Could you check a few things on this model? Use its own coordinates, in mm. Round coordinates to 2 decimals unless told otherwise and drop trailing zeros. Write each loop counter-clockwise with the first axis right and the second up, starting at its lowest first coordinate (ties: lowest second). Pieces come first, ordered by that corner, then holes. Notation, with made-up numbers: (11, 12.5) -> (36, 12.5) arc R20 cw to (36, 19.5) -> close; hole circle Ø11 at (14, -1.5). An arc over 180 degrees is marked (long way). Answer in a Markdown table with one row per item.
from build123d import *

# Parameters (mm, degrees)
END_STOP_SHEET_SKETCH_W                   = 2
END_STOP_SHEET_SKETCH_H                   = 54
END_STOP_SHEET_DEPTH                      = 11
SCREW_END_CLEARANCE_SKETCH_R              = 3.4
SCREW_END_CLEARANCE_DEPTH                 = 2.2
M3_COUNTERSUNK_CLEARANCE_1_BORE_PROFILE_R = 1.7
M3_COUNTERSUNK_CLEARANCE_1_BORE_DEPTH     = 2.2
M3_COUNTERSUNK_CLEARANCE_2_BORE_PROFILE_R = 1.7
M3_COUNTERSUNK_CLEARANCE_2_BORE_DEPTH     = 2.2


with BuildPart() as part:
    # End stop sheet sketch → End stop sheet (new body)
    with BuildSketch(Plane.XY.offset(-33.5)):
        with Locations((59.2, -27.5)):
            Rectangle(END_STOP_SHEET_SKETCH_W, END_STOP_SHEET_SKETCH_H)
    extrude(amount=END_STOP_SHEET_DEPTH)

    # Screw end clearance sketch → Screw end clearance (cut)
    with BuildSketch(Plane(origin=(58.1, 0, 0), x_dir=(0, 0, -1), z_dir=(1, 0, 0))):
        with Locations((19.5, -29)):
            Circle(SCREW_END_CLEARANCE_SKETCH_R)
    extrude(amount=SCREW_END_CLEARANCE_DEPTH, mode=Mode.SUBTRACT)

    # M3 countersunk clearance 1 bore profile → M3 countersunk clearance 1 bore (cut)
    with BuildSketch(Plane.ZY.offset(-60.2)):
        with Locations(Location((-28, -18.5, 0), (0, 0, 180))):
            Circle(M3_COUNTERSUNK_CLEARANCE_1_BORE_PROFILE_R)
    extrude(amount=M3_COUNTERSUNK_CLEARANCE_1_BORE_DEPTH, mode=Mode.SUBTRACT)

    # M3 countersunk clearance 1 countersink p → M3 countersunk clearance 1 countersink (revolve, cut)
    with BuildSketch(Plane.XY.offset(-28), mode=Mode.PRIVATE) as m3_countersunk_clearance_1_countersink_sk:
        Polygon((60.2, -18.5), (60.2, -15.3), (58.7, -16.8), (58.7, -18.5), align=None)
    revolve(m3_countersunk_clearance_1_countersink_sk.sketch.rotate(Axis((70.2, -18.5, -28), (-1, 0, 0)), 90), axis=Axis((70.2, -18.5, -28), (-1, 0, 0)), mode=Mode.SUBTRACT)

    # M3 countersunk clearance 2 bore profile → M3 countersunk clearance 2 bore (cut)
    with BuildSketch(Plane.ZY.offset(-60.2)):
        with Locations(Location((-28, -38.5, 0), (0, 0, 180))):
            Circle(M3_COUNTERSUNK_CLEARANCE_2_BORE_PROFILE_R)
    extrude(amount=M3_COUNTERSUNK_CLEARANCE_2_BORE_DEPTH, mode=Mode.SUBTRACT)

    # M3 countersunk clearance 2 countersink p → M3 countersunk clearance 2 countersink (revolve, cut)
    with BuildSketch(Plane.XY.offset(-28), mode=Mode.PRIVATE) as m3_countersunk_clearance_2_countersink_sk:
        Polygon((60.2, -38.5), (60.2, -35.3), (58.7, -36.8), (58.7, -38.5), align=None)
    revolve(m3_countersunk_clearance_2_countersink_sk.sketch.rotate(Axis((70.2, -38.5, -28), (-1, 0, 0)), 90), axis=Axis((70.2, -38.5, -28), (-1, 0, 0)), mode=Mode.SUBTRACT)


with BuildPart() as body_2:
    # Mirror1: mirrored copy
    add(part.part.mirror(Plane(origin=(0, 0, 0), x_dir=(0, 0, 1), z_dir=(0, -1, 0))))


solid = body_2.part
1) Imagine slicing it at B-B, the plane x = 59.45. Please give me the cut outline in (y, z), plus the area to 3 significant figures.
Findings:
| item | result |
|---|---|
| outline | (0.5, -33.5) -> (54.5, -33.5) -> (54.5, -22.5) -> (30.6, -22.5) arc R3.4 cw to (27.4, -22.5) -> (0.5, -22.5) -> close; hole circle Ø4.9 at (18.5, -28); hole circle Ø4.9 at (38.5, -28) |
| area | 555 mm^2 |
2) Imagine slicing it at A-A, the plane z = -28. Please give me the cut outline in (x, y).
Findings:
| item | result |
|---|---|
| outline | (58.2, 0.5) -> (60.2, 0.5) -> (60.2, 15.3) -> (58.7, 16.8) -> (58.2, 16.8) -> close; (58.2, 20.2) -> (58.7, 20.2) -> (60.2, 21.7) -> (60.2, 35.3) -> (58.7, 36.8) -> (58.2, 36.8) -> close; (58.2, 40.2) -> (58.7, 40.2) -> (60.2, 41.7) -> (60.2, 54.5) -> (58.2, 54.5) -> close |
3) Imagine slicing it at D-D, the plane y = 29. Please give me the cut outline in (x, z), plus the area to 3 significant figures.
Findings:
| item | result |
|---|---|
| outline | (58.2, -33.5) -> (60.2, -33.5) -> (60.2, -22.9) -> (58.2, -22.9) -> close |
| area | 21.2 mm^2 |
4) Please list where these lines run through material, in increasing order: line 1 (Y direction, x = 58.45, z = -28); line 2 (Z direction, x = 58.35, y = 38.5); line 3 (Y direction, x = 60, z = -29.5).
Findings:
| item | result |
|---|---|
| line 1 | y = 0.5 to 16.8, 20.2 to 36.8, 40.2 to 54.5 |
| line 2 | z = -33.5 to -29.7, -26.3 to -22.5 |
| line 3 | y = 0.5 to 15.9, 21.1 to 35.9, 41.1 to 54.5 |
5) For pin 1 (2.5 mm diameter, centred on y = 38.5, z = -28, fed in from -X); pin 2 (5.5 mm diameter, centred on y = 18.5, z = -28, fed in from +X), each with a flat end and sliding along its axis, tell me the tip position at first contact or that it passes through.
Findings:
| item | result |
|---|---|
| pin 1 | passes through |
| pin 2 | stops at x = 59.75 |
6) Thinking about a two-plate mould opening in Y: for faces 1 (the face through (58.5, 37, -28.8)), 2 (the face through (59, 54.5, -28)), 3 (the face through (58.45, 19.01, -29.62)), 4 (the face through (59, 42, -22.5)), which applies, +Y half, -Y half, draft (parallel to the pull), parting line (faces both ways), or undercut?
Findings:
| item | result |
|---|---|
| face 1 | undercut |
| face 2 | +Y half |
| face 3 | undercut |
| face 4 | draft |
7) Imagine slicing it at C-C, the plane y = 38.5. Please give me the cut outline in (x, z).
Findings:
| item | result |
|---|---|
| outline | (58.2, -33.5) -> (60.2, -33.5) -> (60.2, -31.2) -> (58.7, -29.7) -> (58.2, -29.7) -> close; (58.2, -26.3) -> (58.7, -26.3) -> (60.2, -24.8) -> (60.2, -22.5) -> (58.2, -22.5) -> close |
